Geometry: see drawing. Coordinates: mm, zero at the bounding-box minimum. A direction names the side the tool comes from. Coordinates: 2 decimals unless noted, no trailing zeros. Write each loop counter-clockwise with the first axis right and the second up, starting at its lowest first coordinate (ties: lowest second). Pieces come first, ordered by that corner, then holes. Notation, with made-up numbers: (24, 3) - (72, 3) arc R6 cw to (72, 9) - close; hole circle Ø2 at (-39.75, 53). An arc over 180 degrees is marked (long way). Use a Markdown table: item, result. Add a question column.
Q1. Section query D-D (x = 26). Return the cut outline in (y, z).
Q2. Section query B-B (y = 9.5). Return the cut outline in (x, z), then the cut area to 3 significant figures.
Q3. Pin query (flat end, axial travel): P1, Ø6.5, axis at x = 16, z = 11, coming from the -Y side; P2, Ø0.5, axis at x = 31.5, z = 10.5, coming from the +Y side; P3, Ø3, axis at x = 23, y = 23, coming from the +Z side. Return the tip coordinate at first contact, or that it passes through.
Q4. Mould query, pull axis Z, two halves, no side actions, for the marked faces 4, 5, 6 and 7. Classes: released by +Z, released by -Z, zero draft, split by the parting line, or undercut.
Q5. Section query C-C (z = 3.5). Return the cut outline in (x, y).
Q6. Section query A-A (z = 11). Return the cut outline in (x, y).
Q7. Material intervals for probe 1 along Z at (x, y) = (7, 14.5); probe 2 along X at (y, z) = (15.5, 5.5); probe 3 along X at (y, z) = (23.5, 11), sorted ascending. Write a range as from..to.
Q8. Set-up query: the marked faces 1, 2 and 3. Return all of +Z, -Z, +X, -X, +Y, -Y with unobstructed straight access to the full face (end or side cutting, diameter ignored); none if empty.
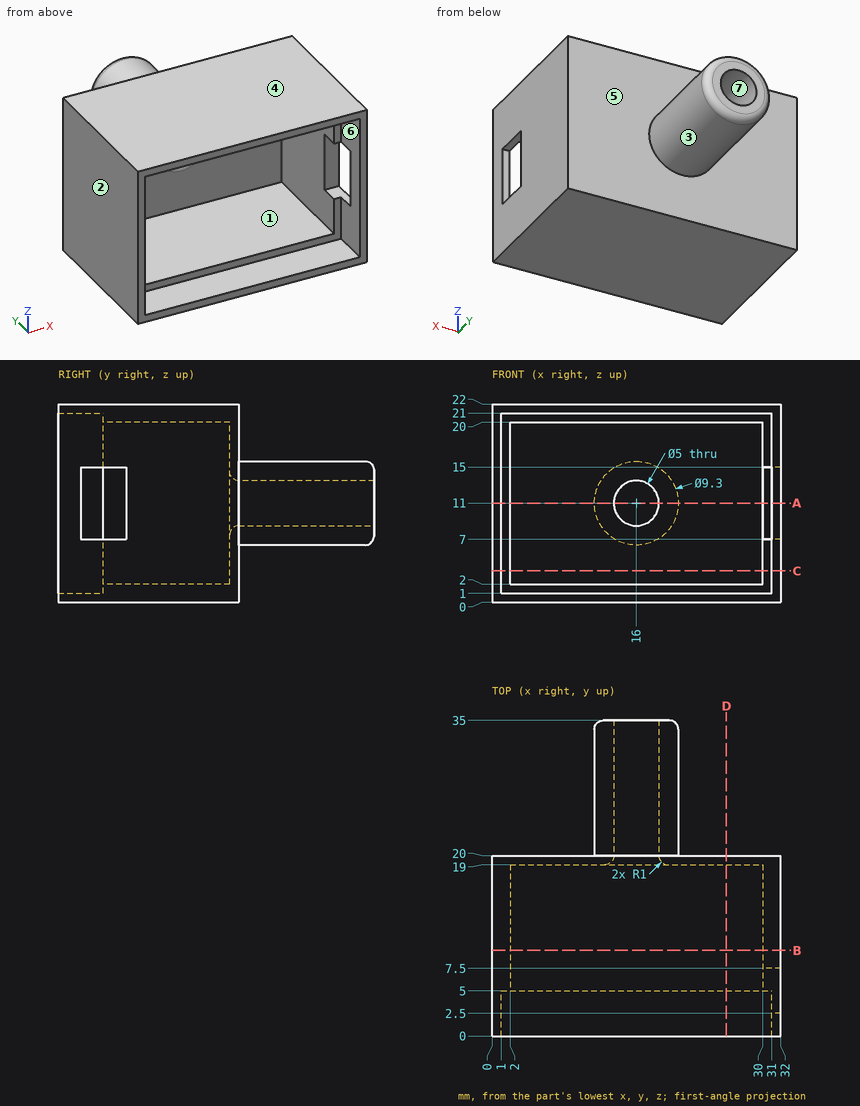
Values follow:
| question | item | result |
|---|---|---|
| 1 | outline | (0, 0) - (20, 0) - (20, 22) - (0, 22) - (0, 21) - (5, 21) - (5, 20) - (19, 20) - (19, 2) - (5, 2) - (5, 1) - (0, 1) - close |
| 2 | outline | (0, 0) - (32, 0) - (32, 22) - (0, 22) - close; hole (2, 2) - (30, 2) - (30, 20) - (2, 20) - close |
| 2 | area | 200 mm2 |
| 3 | P1 | y = 19.03 |
| 3 | P2 | y = 20 |
| 3 | P3 | through |
| 4 | face 4 | released by +Z |
| 4 | face 5 | zero draft |
| 4 | face 6 | undercut |
| 4 | face 7 | undercut |
| 5 | outline | (0, 0) - (1, 0) - (1, 5) - (2, 5) - (2, 19) - (30, 19) - (30, 5) - (31, 5) - (31, 0) - (32, 0) - (32, 20) - (0, 20) - close |
| 6 | outline | (0, 0) - (1, 0) - (1, 5) - (2, 5) - (2, 19) - (12.5, 19) arc R1 ccw to (13.5, 20) - (13.5, 35) - (12.35, 35) arc R1 ccw to (11.35, 34) - (11.35, 20) - (0, 20) - close; (18.5, 20) arc R1 ccw to (19.5, 19) - (30, 19) - (30, 7.5) - (32, 7.5) - (32, 20) - (20.65, 20) - (20.65, 34) arc R1 ccw to (19.65, 35) - (18.5, 35) - close; (31, 0) - (32, 0) - (32, 2.5) - (31, 2.5) - close |
| 7 | probe 1 | 0..2, 20..22 |
| 7 | probe 2 | 0..2, 30..32 |
| 7 | probe 3 | 11.35..13.5, 18.5..20.65 |
| 8 | face 1 | -Y |
| 8 | face 2 | +Z, -Z, -X, +Y, -Y |
| 8 | face 3 | +Y |
